Here's the drawing with two shaded views (mm, measured from the low corner). I have some questions. Coordinates: 2 decimals unless noted, no trailing zeros. Loops run counter-clockwise (first coordinate to the right, second up) from the corner with the lowest first, then second, coordinate; pieces in that order, holes last.
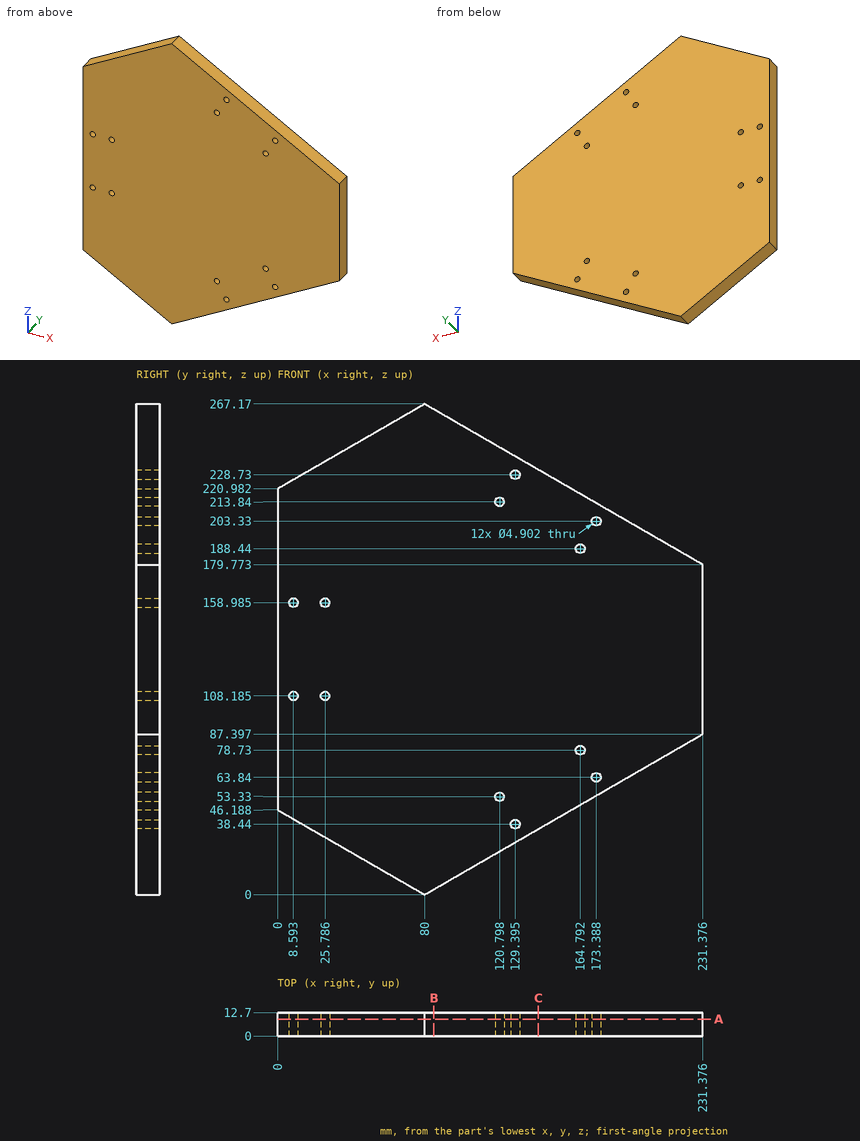
(1) I want a section at C-C on x = 142. Write out the boundary of the cut face in (y, z) (1 decimal), then the cut area to 3 significant figures.
Check values:
outline: (0, 35.8) - (12.7, 35.8) - (12.7, 231.4) - (0, 231.4) - close
area: 2,480 mm2
(2) If I drill on probe 1 along X at (y, z) = (4.75, 52) (1 decimal); probe 2 along Z at (x, y) = (188, 6) (1 decimal); probe 3 along Z at (x, y) = (157, 8) (1 decimal), over which ranges is the centre line in solid material (lowest first)?
Check values:
probe 1: x = 0 to 118.7, 122.9 to 170.1
probe 2: z = 62.4 to 204.8
probe 3: z = 44.5 to 222.7
(3) I'm going to push flat-ended pins straight in: pin 1 (6 mm diameter, centred on y = 7.5, z = 204.5, fed in from +X) (1 decimal); pin 2 (4.5 mm diameter, centred on x = 173.39, z = 63.84, fed in from -Y); pin 3 (3 mm diameter, centred on x = 45.5, y = 3, fed in from +Z); pin 4 (3 mm diameter, centred on y = 3, z = 74, fed in from +X). Where does each tip first touch, or does it pass through?
Check values:
pin 1: stops at x = 193.7
pin 2: passes through
pin 3: stops at z = 248.12
pin 4: stops at x = 210.77
(4) I want a section at B-B on x = 85. Write out the boundary of the cut face in (y, z), then the cut area to 3 significant figures.
Check values:
outline: (0, 2.89) - (12.7, 2.89) - (12.7, 264.28) - (0, 264.28) - close
area: 3,320 mm2
(5) I want a section at A-A on y = 9.25. State how many separate pieces and enclosed holes the cut face has, then the cut area to 3 significant figures.
Check values:
separate pieces: 1
enclosed holes: 12
area: 44,700 mm2
